The drawing under review shows one solid part. Ordinate dimensions are in mm from its lowest x, y, z. A direction names the side the tool comes from. Coordinates: 2 decimals unless noted, no trailing zeros. Write each loop counter-clockwise with the first axis right and the second up, starting at its lowest first coordinate (ties: lowest second). Pieces come first, ordered by that corner, then holes. Notation, with made-up numbers: (32.5, -19.5) - (48.5, -19.5) arc R20 cw to (48.5, 10.5) - close; hole circle Ø1 at (81.25, 38). An arc over 180 degrees is marked (long way). Put each result on its own line as item: value. Start each with the question number.
Item 1: Consider section B-B on y = 420. Give the boundary of the cut face in (x, z).
Item 2: For pin 1 (1 mm diameter, centred on y = 197, z = 194, fed in from -X); pin 2 (2 mm diameter, centred on x = 188.5, z = 109, fed in from -Y); pin 3 (1.5 mm diameter, centred on x = 301.5, z = 191, fed in from +Y), all flat-tipped, find the tip position at first contact; note any pin that passes through.
Item 3: Mouldability with a two-part tool opening along Y and no side actions: class the marked faces 1, 2, 3 and 4 as pulls with the +Y half, pulls with the -Y half, needs draft (parallel to the pull), parting line crosses it, or undercut.
Item 4: Consider section A-A on y = 225. Give the boundary of the cut face in (x, z).
Item 5: Consider section D-D on z = 164.5. Give the boundary of the cut face in (x, y), then the cut area to 3 significant figures.
Item 6: Consider section C-C on x = 400. Give the boundary of the cut face in (y, z), then the cut area to 3 significant figures.
Item 7: Machinability: for the marked faces 5 and 6, which of the approach directions +Z, -Z, +X, -X, +Y, -Y give a long, thin tool a straight path to every point of the face, cutting with its end or side? Answer none if there is none.
Item 8: To check wall thickness, follow L1, parallel to Y at x = 225, z = 180; L2, parallel to Z at x = 353.5, y = 244; L3, parallel to X at y = 246, z = 172.5. State the ranges of each line that lie inside material, in increasing order. Write a range as [from, to].
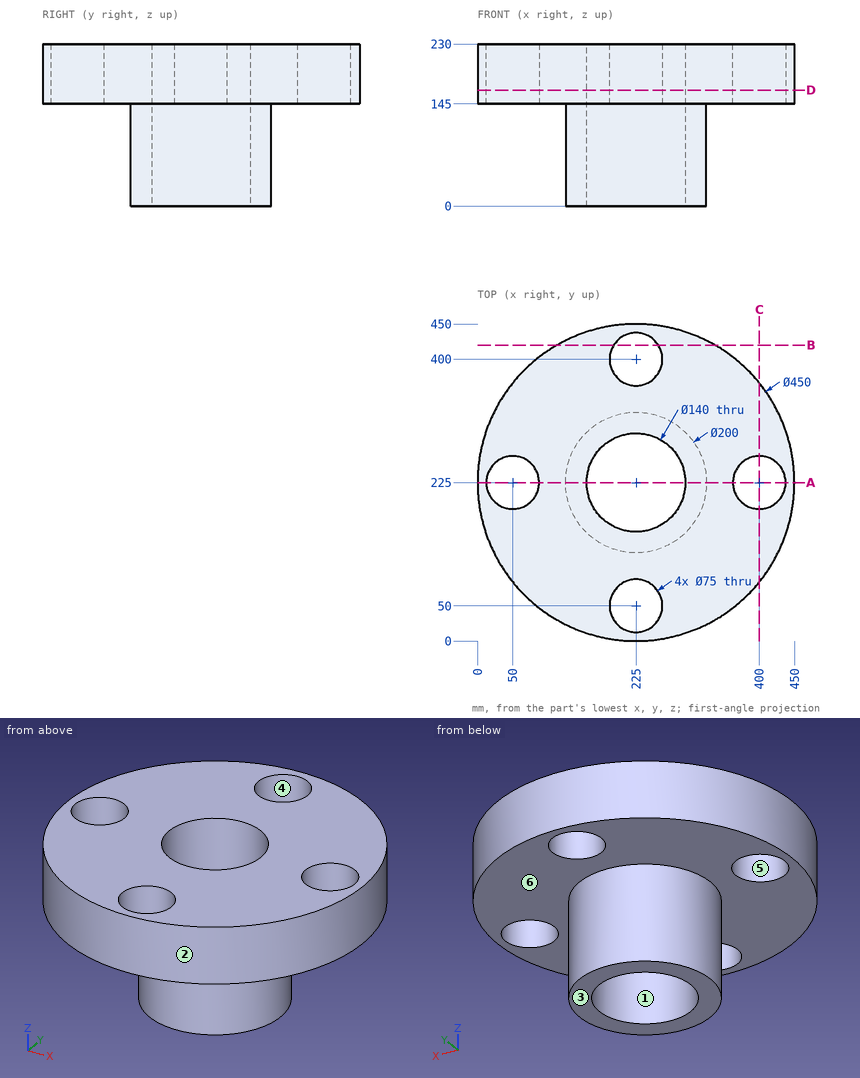
Report:
1. outline: (112.75, 145) - (193.28, 145) - (193.28, 230) - (112.75, 230) - close; (256.72, 145) - (337.25, 145) - (337.25, 230) - (256.72, 230) - close
2. pin 1: x = 1.69
2. pin 2: y = 131.51
2. pin 3: y = 436.87
3. face 1: undercut
3. face 2: parting line crosses it
3. face 3: needs draft
3. face 4: undercut
4. outline: (0, 145) - (12.5, 145) - (12.5, 230) - (0, 230) - close; (87.5, 145) - (125, 145) - (125, 0) - (155, 0) - (155, 230) - (87.5, 230) - close; (295, 0) - (325, 0) - (325, 145) - (362.5, 145) - (362.5, 230) - (295, 230) - close; (437.5, 145) - (450, 145) - (450, 230) - (437.5, 230) - close
5. outline: circle Ø450 at (225, 225); hole circle Ø75 at (50, 225); hole circle Ø140 at (225, 225); hole circle Ø75 at (225, 50); hole circle Ø75 at (225, 400); hole circle Ø75 at (400, 225)
5. area: 126,000 mm²
6. outline: (83.58, 145) - (187.5, 145) - (187.5, 230) - (83.58, 230) - close; (262.5, 145) - (366.42, 145) - (366.42, 230) - (262.5, 230) - close
6. area: 17,700 mm²
7. face 5: +Z, -Z
7. face 6: -Z
8. L1: [0, 12.5], [87.5, 155], [295, 362.5], [437.5, 450]
8. L2: [145, 230]
8. L3: [0.98, 18.93], [81.07, 158.22], [291.78, 368.93], [431.07, 449.02]
